from build123d import *

# Parameters (mm, degrees)
SKETCH1_W           = 30
SKETCH1_H           = 32
BOSS_EXTRUDE1_DEPTH = 6.5
CUT_EXTRUDE1_REACH  = 46.342
SKETCH2_W           = 11.5
SKETCH2_H           = 26


with BuildPart() as part:
    # Sketch1 → Boss-Extrude1 (new body)
    with BuildSketch(Plane.XY):
        with Locations((15, 16)):
            Rectangle(SKETCH1_W, SKETCH1_H)
    extrude(amount=BOSS_EXTRUDE1_DEPTH)

    # Sketch2 → Cut-Extrude1 (cut, up to next)
    with BuildSketch(Plane.XY.offset(6.5), mode=Mode.PRIVATE) as cut_extrude1_sk1:
        with Locations((5.75, 13)):
            Rectangle(SKETCH2_W, SKETCH2_H)
    cut_extrude1_tool1 = extrude(cut_extrude1_sk1.sketch, amount=-CUT_EXTRUDE1_REACH, mode=Mode.PRIVATE) & part.part
    # Sketch2 → Cut-Extrude1 (cut, up to next)
    with BuildSketch(Plane.XY.offset(6.5), mode=Mode.PRIVATE) as cut_extrude1_sk2:
        with Locations((24.25, 13)):
            Rectangle(SKETCH2_W, SKETCH2_H)
    cut_extrude1_tool2 = extrude(cut_extrude1_sk2.sketch, amount=-CUT_EXTRUDE1_REACH, mode=Mode.PRIVATE) & part.part
    add(cut_extrude1_tool1.solids().sort_by_distance((5.75, 13, 6.5))[0], mode=Mode.SUBTRACT)
    add(cut_extrude1_tool2.solids().sort_by_distance((24.25, 13, 6.5))[0], mode=Mode.SUBTRACT)


solid = part.part
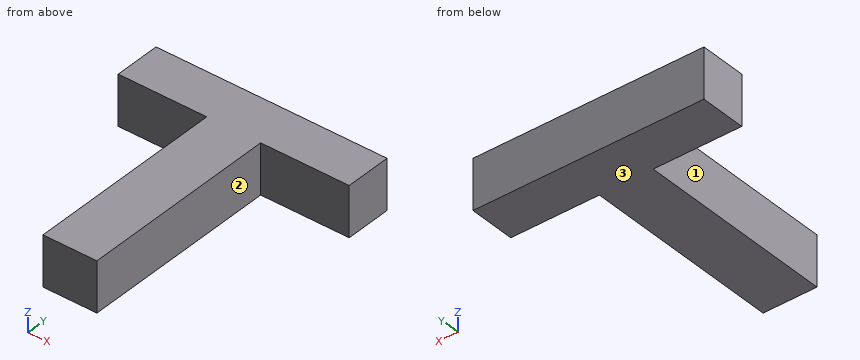
Here's how the part is built. I have some questions about the finished solid (model axes, mm). Face numbers are marked on the shaded views. A direction names the side the tool comes from. Round coordinates to 2 decimals unless told otherwise and drop trailing zeros. Loops run counter-clockwise (first coordinate to the right, second up) from the corner with the lowest first, then second, coordinate; pieces in that order, holes last. Notation, with made-up numbers: (74, -10) - (101, -10) arc R28 ccw to (101, 27) - close; hole circle Ø11 at (80, 36.25). An arc over 180 degrees is marked (long way). One line per question, with ' | ' between items. Start each with the question number.
Q1. I want a section at B-B (y = 7). Write out the boundary of the cut face in (x, z), then the cut area to 3 significant figures.
Q2. Please list where these lines run through material, in increasing order: line 1 (X direction, y = 21, z = 2.75); line 2 (Y direction, x = 19.25, z = 3.25). Write a range as [from, to].
Q3. I want a section at C-C (x = 5.25). Write out the boundary of the cut face in (y, z).
Q4. Will these pins go through, and if not, where does the flat tip stop? pin 1 (3 mm diameter, centred on x = 20.5, z = 1.5, fed in from -Y); pin 2 (3 mm diameter, centred on y = 5, z = 5, fed in from -X); pin 3 (3 mm diameter, centred on y = 10, z = 3, fed in from +X).
Q5. I want a section at A-A (z = 0.75). Write out the boundary of the cut face in (x, y), then the cut area to 3 significant figures.
Q6. For the marked faces 1, 2 and 3, which set-ups out of +Z, -Z, +X, -X, +Y, -Y let a thin tool reach every point of the face, with its end or its side?
Response values:
1) outline: (11.5, 0) - (18.5, 0) - (18.5, 6.5) - (11.5, 6.5) - close | area: 45.5 mm²
2) line 1: x = [11.5, 18.5] | line 2: y = [26, 32]
3) outline: (26, 0) - (32, 0) - (32, 6.5) - (26, 6.5) - close
4) pin 1: stops at y = 26 | pin 2: stops at x = 11.5 | pin 3: stops at x = 18.5
5) outline: (0, 26) - (11.5, 26) - (11.5, 0) - (18.5, 0) - (18.5, 26) - (30, 26) - (30, 32) - (0, 32) - close | area: 362 mm²
6) face 1: +Z, -Z, -X, -Y | face 2: +Z, -Z, +X, -Y | face 3: -Z, +X, -X, +Y, -Y
